Check sheet for the drawn part. Datum: minimum x, y, z corner. Units: mm. A direction names the side the tool comes from. Round coordinates to 2 decimals unless told otherwise and drop trailing zeros. Write each loop counter-clockwise with the first axis right and the second up, starting at its lowest first coordinate (ties: lowest second). Pieces come first, ordered by that corner, then holes. Notation, with made-up numbers: (2, 82) - (20, 82) arc R15 ccw to (20, 106) - close; hole circle Ø11 at (79.25, -37.5). An arc over 180 degrees is marked (long way). Answer as a JSON object with one key per item and string values.
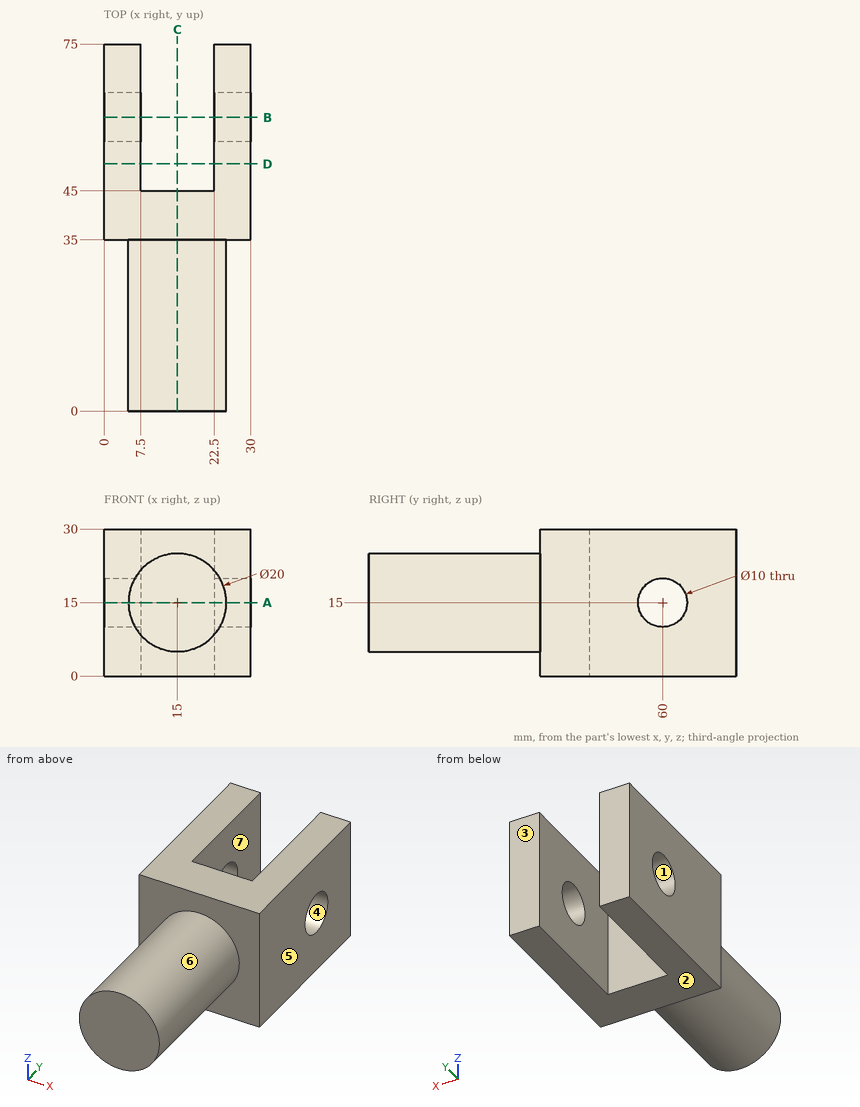
Q1. Section check B-B, the plane y = 60. Record the cut outline in (x, z), then the cut area to 3 significant figures.
Geometry check:
{"outline": "(0, 0) - (7.5, 0) - (7.5, 10) - (0, 10) - close; (0, 20) - (7.5, 20) - (7.5, 30) - (0, 30) - close; (22.5, 0) - (30, 0) - (30, 10) - (22.5, 10) - close; (22.5, 20) - (30, 20) - (30, 30) - (22.5, 30) - close", "area": "300 mm2"}
Q2. Section check C-C, the plane x = 15. Record the cut outline in (y, z).
Geometry check:
{"outline": "(0, 5) - (35, 5) - (35, 0) - (45, 0) - (45, 30) - (35, 30) - (35, 25) - (0, 25) - close"}
Q3. Gauge pin test, flat end, axial feed: P1, Ø1.5, axis at x = 8.5, z = 25.5, coming from the +Y side. Record the tip position at first contact, or that the pin passes through.
Geometry check:
{"P1": "stops at y = 45"}
Q4. Section check D-D, the plane y = 50.5. Record the cut outline in (x, z), then the cut area to 3 significant figures.
Geometry check:
{"outline": "(0, 0) - (7.5, 0) - (7.5, 30) - (0, 30) - close; (22.5, 0) - (30, 0) - (30, 30) - (22.5, 30) - close", "area": "450 mm2"}
Q5. Material ranges on line 1 along X through (y, z) = (50, 19.75); line 2 along Y through (x, z) = (24.5, 15); line 3 along Y through (x, z) = (21, 20.75), recorded low to high. Write a range as [from, to].
Geometry check:
{"line 1": "x = [0, 7.5], [22.5, 30]", "line 2": "y = [0, 55], [65, 75]", "line 3": "y = [0, 45]"}
Q6. Set-up check for the marked faces 5, 6 and 7: record each of +Z, -Z, +X, -X, +Y, -Y from which the full face is reachable in a straight line by a thin tool's end or side.
Geometry check:
{"face 5": "+Z, -Z, +X, +Y, -Y", "face 6": "-Y", "face 7": "+Z, -Z, +Y"}
Q7. Section check A-A, the plane z = 15. Record the cut outline in (x, y).
Geometry check:
{"outline": "(0, 35) - (5, 35) - (5, 0) - (25, 0) - (25, 35) - (30, 35) - (30, 55) - (22.5, 55) - (22.5, 45) - (7.5, 45) - (7.5, 55) - (0, 55) - close; (0, 65) - (7.5, 65) - (7.5, 75) - (0, 75) - close; (22.5, 65) - (30, 65) - (30, 75) - (22.5, 75) - close"}
Q8. Release check for a two-part mould opening along Z. For the marked faces 1, 2, 3 and 4 record: released by +Z, released by -Z, zero draft, split by the parting line, or undercut.
Geometry check:
{"face 1": "undercut", "face 2": "released by -Z", "face 3": "zero draft", "face 4": "undercut"}
